Check sheet for the modelled part. Datum: model origin and axes. Units: mm. A direction names the side the tool comes from. Give positions to 0.01 mm unless a question says otherwise; leave off trailing zeros. Loops run counter-clockwise (first coordinate to the right, second up) from the corner with the lowest first, then second, coordinate; pieces in that order, holes last. Notation, with made-up numbers: M 0.5,-24.5 L 14.5,-24.5 A25 cw 14.5,8.5 Z; hole C -30,35 d7. An arc over 180 degrees is marked long. One line per question, with ' | ' between items. Start each with the question number.
from build123d import *

# Parameters (mm, degrees)
CUT_EXTRUDE1_DEPTH = 172.951680952


with BuildPart() as part:
    # Sketch1 → Revolve1 (revolve)
    with BuildSketch(Plane.XY, mode=Mode.PRIVATE) as revolve1_sk:
        with BuildLine():
            Line((0, -76.2), (53.76994832, -76.2))
            ThreePointArc((53.76994832, -76.2), (56.183319637, -74.451984147), (55.274949756, -71.613888889))
            ThreePointArc((55.274949756, -71.613888889), (19.05, 0), (55.274949756, 71.613888889))
            ThreePointArc((55.274949756, 71.613888889), (56.183319637, 74.451984147), (53.76994832, 76.2))
            Line((53.76994832, 76.2), (0, 76.2))
            Line((0, 76.2), (0, -76.2))
        make_face()
    revolve(revolve1_sk.sketch.rotate(Axis((0, -76.2, 0), (0, 1, 0)), 90), axis=Axis((0, -76.2, 0), (0, 1, 0)))

    # Sketch3 → Cut-Extrude1 (cut, through all)
    with BuildSketch(Plane(origin=(0, 76.2, 0), x_dir=(1, 0, 0), z_dir=(0, 1, 0))):
        Polygon((7.405671903, 0), (3.702835951, -6.4135), (-3.702835951, -6.4135), (-7.405671903, 0), (-3.702835951, 6.4135), (3.702835951, 6.4135), align=None)
    extrude(amount=-CUT_EXTRUDE1_DEPTH, mode=Mode.SUBTRACT)


solid = part.part
Q1. Draft check along X on faces 3 (the flat face through (5.5, 1.1, -3.3)), 4 (the flat face through (0, 1, -6.414)), 5 (the flat face through (-1, 76.2, -11)). Enter one of: released by +X, released by -X, zero draft, split by the parting line, or undercut.
Q2. Depth check by flat-ended pin: P1, Ø6, axis at x = 0, y = 26, coming from the +Z side; P2, Ø8, axis at x = 27, y = 19, coming from the +Z side; P3, Ø3, axis at x = 26.5, y = -43, coming from the -Z side; P4, Ø10, axis at y = -32.5, z = -26.5, coming from the -X side. Enter the tip coordinate at first touch or a pass-through.
Q3. Cross-section at B-B (y = 58). Record the cut outline in (x, z), and give its area (3 significant figures).
Q4. Cross-section at A-A (y = 7). Record the cut outline in (x, z), and give its area (3 significant figures).
Q5. Material ranges on probe 1 along Y at (x, z) = (11.5, 32); probe 2 along Y at (x, z) = (-40, 10); probe 3 along Z at (x, y) = (10.5, 20), recorded low to high. Write a range as from..to.
Q6. Access from +Z, -Z, +X, -X, +Y, -Y to the whole of each face (thin tool, end or side, straight path). Record for faces 1 (the flat face through (5.58, 1.07, 3.16)), 2 (the flat face through (-1, -76.2, 11)).
Solved:
1) face 3: undercut | face 4: undercut | face 5: zero draft
2) P1: stops at z = 23.91 | P2: passes through | P3: stops at z = -17.3 | P4: stops at x = -14.03
3) outline: C 0,0 d81.15; hole M -7.41,0 L -3.7,-6.41 L 3.7,-6.41 L 7.41,0 L 3.7,6.41 L -3.7,6.41 Z | area: 5,030 mm²
4) outline: C 0,0 d38.65; hole M -7.41,0 L -3.7,-6.41 L 3.7,-6.41 L 7.41,0 L 3.7,6.41 L -3.7,6.41 Z | area: 1,030 mm²
5) probe 1: y = -76.2..-49.35, 49.35..76.2 | probe 2: y = -76.2..-58.75, 58.75..76.2 | probe 3: z = -18.57..18.57
6) face 1: +Y, -Y | face 2: +Z, -Z, +X, -X, -Y
